Design review of the part shown in the three views and the two pictorial views. Dimensions are in mm from the part's minimum x, y and z. Give positions to 0.01 mm unless a question says otherwise; leave off trailing zeros. Loops run counter-clockwise (first coordinate to the right, second up) from the corner with the lowest first, then second, coordinate; pieces in that order, holes last. Notation, with made-up numbers: (32.25, 16) -> (84.25, 16) arc R21 ccw to (84.25, 45) -> close; hole circle Ø10 at (-9, 56.5). An arc over 180 degrees is marked (long way). Use CSV: the item, a comma, the result in double quotes. Start each with the question number.
Item 1: Wall thickness on line 1 along X through (y, z) = (186, 658); line 2 along Z through (x, y) = (265, 238); line 3 along Z through (x, y) = (32, 352) (1 decimal): over which ranges is each line inside the solid? List them lowest first. Write a range as from..to.
Item 2: We need section A-A (x = 137). State the section outline as (y, z) points.
Item 3: The part is to be moulded in two halves that separate along Z. For the marked faces 1 and 2, say which applies: +Z half, -Z half, draft (parallel to the pull), parting line (faces both ways), or undercut.
Item 4: Clearance check with flat-ended pins moving along their axes: pin 1 (2 mm diameter, centred on x = 212, z = 367.5, fed in from +Y); pin 2 (4 mm diameter, centred on x = 192, z = 589, fed in from -Y); pin 3 (3 mm diameter, centred on x = 332, z = 582.5, fed in from -Y). State where each tip first meets the part, or that it passes through.
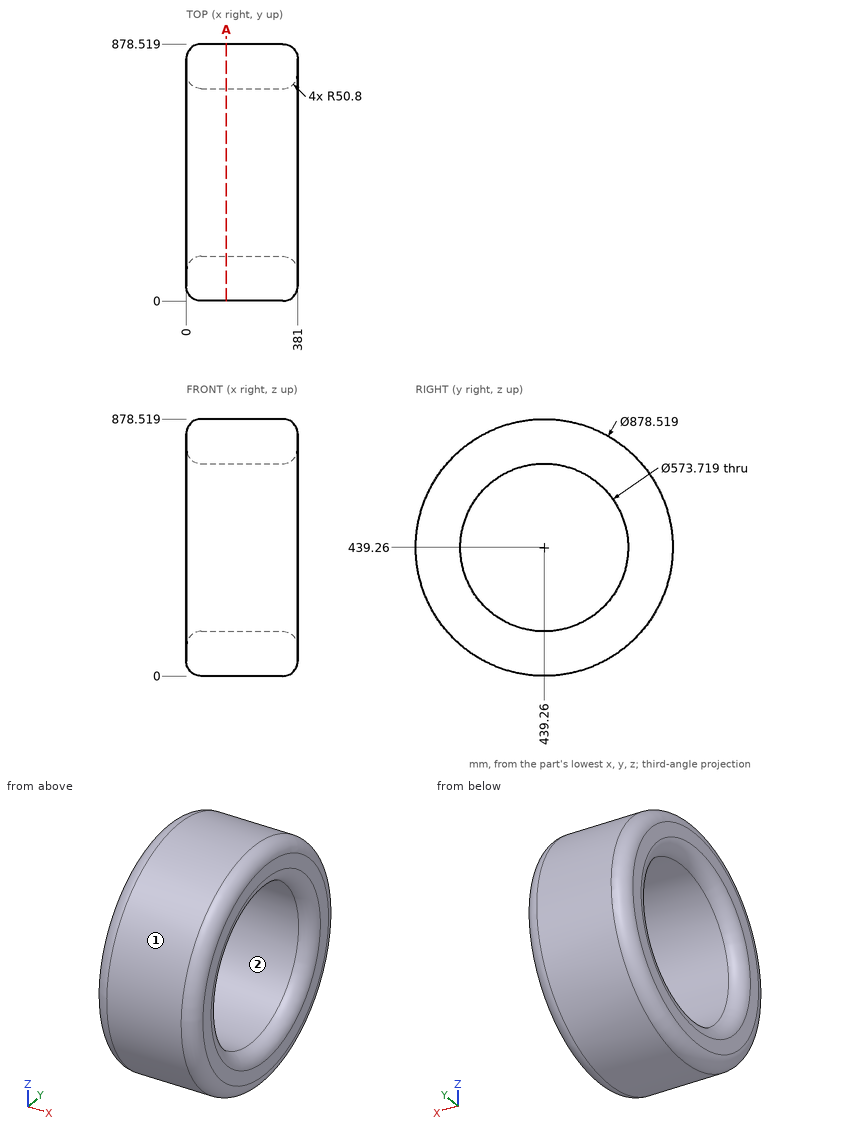
Results found:
1,line 1,"0.09..380.91"
1,line 2,"48.82..234.85, 643.67..829.7"
1,line 3,"12.4..162.2, 716.3..866.1"
2,outline,"circle Ø878.52 at (439.26, 439.26); hole circle Ø573.72 at (439.26, 439.26)"
3,face 1,"parting line"
3,face 2,"undercut"
4,pin 1,"y = 872.78"
4,pin 2,"y = 25.59"
4,pin 3,"y = 23.53"
